Answer from the drawing. Dimensions are ordinates in mm from the lowest x, y and z of the part. Round coordinates to 2 decimals unless told otherwise and drop trailing zeros. Loops run counter-clockwise (first coordinate to the right, second up) from the corner with the lowest first, then second, coordinate; pieces in that order, holes last. Notation, with made-up numbers: (29.5, 4) - (75.5, 4) arc R20 cw to (75.5, 13) - close; hole circle Ø3 at (-3.75, 27). An arc over 180 degrees is marked (long way). Write item = value, one per line. Start each with the question number.
1) Section B-B, the plane x = 74.5 is taken. Determine the outline of the cut face in (y, z).
2) Section A-A, the plane y = 1.85 is taken. Determine the outline of the cut face in (x, z).
3) Given pin 1 Ø1.5 at (y, z) = (2.5, 79) entering from +X, flat-ended and moving along its own axis, determine where the tip first touches the part or whether it passes through.
4) Straight lines are drawn through the part: line 1 along X through (y, z) = (1.8, 138); line 2 along Z through (x, y) = (72.5, 2.5); line 3 along X through (y, z) = (2.1, 33). For each, find the intervals that lie inside material, in ascending order.
5) Section C-C, the plane x = 136 is taken. Determine the outline of the cut face in (y, z), and give its area (3 significant figures).
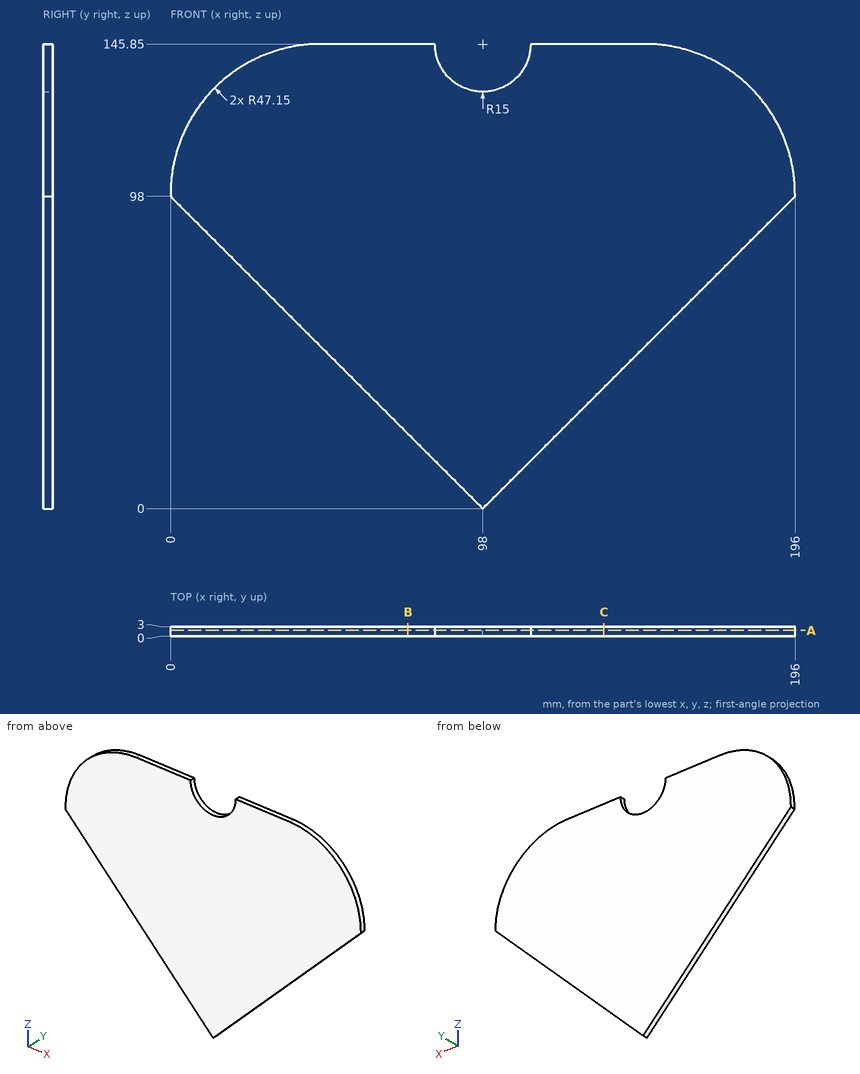
Geometry check:
q1.outline = (0, 23.5) - (3, 23.5) - (3, 145.85) - (0, 145.85) - close
q2.outline = (0, 98) - (98, 0) - (196, 98) - (196, 98.7) arc R47.15 ccw to (148.85, 145.85) - (113, 145.85) arc R15 cw to (83, 145.85) - (47.15, 145.85) arc R47.15 ccw to (0, 98.7) - close
q3.pin_1 = 177.75
q4.line_1 = 21.1 to 85.22, 110.78 to 174.9
q4.line_2 = 25.5 to 145.85
q4.line_3 = 65 to 131
q5.outline = (0, 38) - (3, 38) - (3, 145.85) - (0, 145.85) - close
q5.area = 324 mm2
